```python
from build123d import *

# Parameters (mm, degrees)
SURFACE_EXTRUDE4_1_BACK  = 5
SURFACE_EXTRUDE4_1_DEPTH = 12
THICKEN3_T1              = 2
FILLET3_R                = 0.5


with BuildPart() as body_1:
    # Surface-Extrude4: a surface, the sketch's curves swept straight by 12 mm
    with BuildLine(Plane.XY.offset(-SURFACE_EXTRUDE4_1_BACK), mode=Mode.PRIVATE) as surface_extrude4_1_path:
        Line((-3.067605851, -6.646088585), (-109.286177334, 42.380749855))
        ThreePointArc((-109.286177334, 42.380749855), (-116.178200525, 63.164846887), (-94.987263263, 68.680538237))
        Line((-94.987263263, 68.680538237), (3.910153467, 6.188004445))
        ThreePointArc((3.910153467, 6.188004445), (6.430859787, -3.496389787), (-3.067605851, -6.646088585))
    surface_extrude4_1 = Shell.extrude(surface_extrude4_1_path.wire(), (0 * SURFACE_EXTRUDE4_1_DEPTH, 0 * SURFACE_EXTRUDE4_1_DEPTH, 1 * SURFACE_EXTRUDE4_1_DEPTH))
    add(Solid.thicken(surface_extrude4_1, THICKEN3_T1))

    # Fillet3
    fillet3_edges = [body_1.edges().sort_by_distance(p)[0] for p in [
        (6.430859787, -3.496389787, -5),
        (-56.176891592, 17.867330635, -5),
        (-116.178200525, 63.164846887, -5),
        (-45.538554898, 37.434271341, -5),
        (8.18795319, -4.451702705, 7),
        (-57.01504857, 16.051430615, 7),
        (-117.935293928, 64.120159806, 7),
        (-44.47019, 39.125009772, 7),
        (8.18795319, -4.451702705, -5),
        (-57.01504857, 16.051430615, -5),
        (-117.935293928, 64.120159806, -5),
        (-44.47019, 39.125009772, -5),
        (-45.538554898, 37.434271341, 7),
        (-116.178200525, 63.164846887, 7),
        (-56.176891592, 17.867330635, 7),
        (6.430859787, -3.496389787, 7),
    ]]
    fillet(fillet3_edges, radius=FILLET3_R)


solid = body_1.part
```
Could you check a few things on this model? Use its own coordinates, in mm. A direction names the side the tool comes from. Give positions to 0.01 mm unless a question says otherwise; leave off trailing zeros. Loops run counter-clockwise (first coordinate to the right, second up) from the corner with the lowest first, then second, coordinate; pieces in that order, holes last. Notation, with made-up numbers: (13, -16.5) - (39, -16.5) arc R21 ccw to (39, -11.5) - close; hole circle Ø4 at (8.5, -9). An arc over 180 degrees is marked (long way). Answer in a Markdown table with one row per item. Add a question column.
Q1. If we section it at A-A (z = 3.75): List the corners of the cut face in (x, y) for me.
Q2. For pin 1 (1.5 mm diameter, centred on x = -73, z = 3, fed in from -Y); pin 2 (5 mm diameter, centred on x = -47.5, z = 3.5, fed in from +Y); pin 3 (1 mm diameter, centred on x = -95.5, z = -1.5, fed in from -Y); pin 4 (4 mm diameter, centred on x = -106, y = 42.5, fed in from +Z), each with a flat end and sliding along its axis, tell me the tip position at first contact or that it passes through.
Q3. Please list where these lines run through material, in increasing order: L1, parallel to X at y = 40, z = -3.75; L2, parallel to Y at x = -34, z = 4; L3, parallel to Y at x = -40, z = 3.75. Write a range as from..to.
Q4. Which directions (+Z, -Z, +X, -X, +Y, -Y) give clear straight access to the entire face, cutting with the end or side of a thin tool? Please do faces 4 (the face through (-44.77, 37.12, -4.85)), 5 (the face through (-56.98, 18.08, 6.85)), 6 (the face through (-46.23, 37.87, 0.92)).
Q5. We'd pull the mould along X, two halves only. Please class faces 1 (the face through (-44.77, 37.12, 6.85)), 2 (the face through (-43.854, 38.567, -4.85)), 3 (the face through (-70, 23, -5)): +X half, -X half, draft (parallel to the pull), parting line (faces both ways), or undercut.
The answers:
| question | item | result |
|---|---|---|
| 1 | outline | (-110.12, 40.56) - (-3.91, -8.46) arc R9.32 ccw to (4.98, 7.88) - (-93.92, 70.37) arc R17 ccw (long way) to start; hole (-109.29, 42.38) - (-3.07, -6.65) arc R7.32 ccw to (3.91, 6.19) - (-94.99, 68.68) arc R15 ccw (long way) to start |
| 2 | pin 1 | stops at y = 23.08 |
| 2 | pin 2 | stops at y = 42.62 |
| 2 | pin 3 | stops at y = 33.58 |
| 2 | pin 4 | stops at z = 7 |
| 3 | L1 | x = -108.9..-104.13, -49.6..-45.85 |
| 3 | L2 | y = 5.43..7.63, 30.14..32.51 |
| 3 | L3 | y = 8.2..10.4, 33.93..36.3 |
| 4 | face 4 | -Z |
| 4 | face 5 | +Z |
| 4 | face 6 | +Z, -Z |
| 5 | face 1 | undercut |
| 5 | face 2 | +X half |
| 5 | face 3 | draft |
